Could you check a few things on this model? Use its own coordinates, in mm. Face numbers are marked on the shaded views. A direction names the side the tool comes from. Round coordinates to 2 decimals unless told otherwise and drop trailing zeros. Order: outer loops, then holes, each group sorted by start corner. A loop starts at its lowest first (then second) coordinate and runs counter-clockwise, first axis right, second up. Notation, with made-up numbers: (2, 34.5) - (43, 34.5) arc R32 cw to (43, 72.5) - close; hole circle Ø6 at (-2, 84). An arc over 180 degrees is marked (long way). Use one line per item in the form item = value.
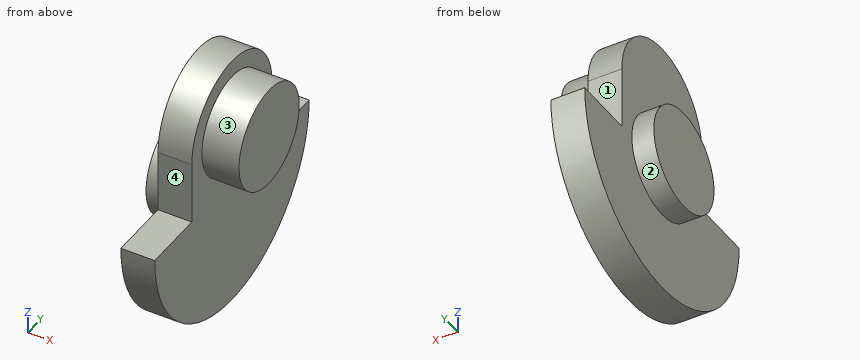
from build123d import *

# Parameters (mm, degrees)
F1_DEPTH  = 2.54
F2_R      = 3.81
F3_DEPTH  = 2.794
F4_R      = 3.81
F5_DEPTH  = 1.5621
F5_FACE_R = 3.81
F6_DEPTH  = 0.0889


with BuildPart() as f1:
    # F0 (on Right) → F1 (new body)
    with BuildSketch(Plane.YZ):
        with BuildLine():
            Line((5.08, 0), (5.08, 4.699))
            ThreePointArc((5.08, 4.699), (0, 9.779), (-5.08, 4.699))
            Line((-5.08, 4.699), (-5.08, 0))
            Line((-5.08, 0), (-9.779, 0))
            ThreePointArc((-9.779, 0), (0, -9.779), (9.779, 0))
            Line((9.779, 0), (5.08, 0))
        make_face()
    extrude(amount=F1_DEPTH)

    # F2 (on face) → F3 (join)
    with BuildSketch(Plane.YZ.offset(2.54)):
        with Locations((0, 4.699)):
            Circle(F2_R)
    extrude(amount=F3_DEPTH)

    # F4 (on face) → F5 (join)
    with BuildSketch(Plane(origin=(0, 0, 0), x_dir=(0, -1, 0), z_dir=(-1, 0, 0))):
        Circle(F4_R)
    extrude(amount=F5_DEPTH)

    # F5_face (on face) → F6 (join)
    with BuildSketch(Plane(origin=(-1.5621, 0, 0), x_dir=(0, -1, 0), z_dir=(-1, 0, 0))):
        Circle(F5_FACE_R)
    extrude(amount=F6_DEPTH)


solid = f1.part
Item 1: Imagine slicing it at A-A on y = 0. Please give me the cut outline in (x, z).
Found:
outline = (-1.65, -3.81) - (0, -3.81) - (0, -9.78) - (2.54, -9.78) - (2.54, 0.89) - (5.33, 0.89) - (5.33, 8.51) - (2.54, 8.51) - (2.54, 9.78) - (0, 9.78) - (0, 3.81) - (-1.65, 3.81) - close
Item 2: Will these pins go through, and if not, where does the flat tip stop? P1, Ø4, axis at x = 3.5, z = 6.5, coming from the -Y side; P2, Ø1.5, axis at x = 0, y = 2, coming from the +Z side; P3, Ø6, axis at y = 4, z = 1.5, coming from the +X side; P4, Ø4, axis at y = -7, z = 7.5, coming from the -X side.
Found:
P1 = -5.08
P2 = 9.62
P3 = 5.33
P4 = through
Item 3: For the marked faces 1, 2, 3 and 4, which set-ups out of +Z, -Z, +X, -X, +Y, -Y let a thin tool reach every point of the face, with its end or its side?
Found:
face_1 = +Z, +X, -X, +Y
face_2 = -X
face_3 = +X
face_4 = +Z, +X, -X, -Y
Item 4: Imagine slicing it at B-B on z = 7.75. Please give me the cut outline in (x, y).
Found:
outline = (0, -4.06) - (2.54, -4.06) - (2.54, -2.28) - (5.33, -2.28) - (5.33, 2.28) - (2.54, 2.28) - (2.54, 4.06) - (0, 4.06) - close
Item 5: Imagine slicing it at D-D on y = -3.5. Please give me the cut outline in (x, z).
Found:
outline = (-1.65, -1.51) - (0, -1.51) - (0, -9.13) - (2.54, -9.13) - (2.54, 3.19) - (5.33, 3.19) - (5.33, 6.2) - (2.54, 6.2) - (2.54, 8.38) - (0, 8.38) - (0, 1.51) - (-1.65, 1.51) - close
Item 6: I need wall thicknesses on L1, parallel to X at y = 9.25, z = -0.25; L2, parallel to Y at x = 0.5, z = 1; L3, parallel to Z at x = 0.75, y = 0. Which ranges of each line are inside material? Lowest first, please.
Found:
L1 = 0 to 2.54
L2 = -5.08 to 5.08
L3 = -9.78 to 9.78
Item 7: Imagine slicing it at C-C on x = 0.25. Please give me the cut outline in (y, z), plus the area to 3 significant figures.
Found:
outline = (-9.78, 0) arc R9.78 ccw to (9.78, 0) - (5.08, 0) - (5.08, 4.7) arc R5.08 ccw to (-5.08, 4.7) - (-5.08, 0) - close
area = 238 mm2
